from build123d import *

# Parameters (mm, degrees)
F1_DEPTH = 2.54
F2_W     = 10.16
F2_H     = 10.16
F3_DEPTH = 2.54


with BuildPart() as f1:
    # F0 (on Top) → F1 (new body)
    with BuildSketch(Plane.XY):
        with BuildLine():
            Line((206.375, -73.81875), (206.375, 73.81875))
            ThreePointArc((206.375, 73.81875), (196.145704, 98.514454), (171.45, 108.74375))
            Line((171.45, 108.74375), (-171.45, 108.74375))
            ThreePointArc((-171.45, 108.74375), (-196.145704, 98.514454), (-206.375, 73.81875))
            Line((-206.375, 73.81875), (-206.375, -73.81875))
            ThreePointArc((-206.375, -73.81875), (-196.145704, -98.514454), (-171.45, -108.74375))
            Line((-171.45, -108.74375), (171.45, -108.74375))
            ThreePointArc((171.45, -108.74375), (196.145704, -98.514454), (206.375, -73.81875))
        make_face()
        with BuildLine():
            ThreePointArc((187.325, -73.81875), (182.67532, -85.04407), (171.45, -89.69375))
            Line((171.45, -89.69375), (-171.45, -89.69375))
            ThreePointArc((-171.45, -89.69375), (-182.67532, -85.04407), (-187.325, -73.81875))
            Line((-187.325, -73.81875), (-187.325, 73.81875))
            ThreePointArc((-187.325, 73.81875), (-182.67532, 85.04407), (-171.45, 89.69375))
            Line((-171.45, 89.69375), (171.45, 89.69375))
            ThreePointArc((171.45, 89.69375), (182.67532, 85.04407), (187.325, 73.81875))
            Line((187.325, 73.81875), (187.325, -73.81875))
        make_face(mode=Mode.SUBTRACT)
    extrude(amount=F1_DEPTH)

    # F2 (on face) → F3 (cut, through all)
    with BuildSketch(Plane.XY.offset(2.54)):
        with Locations((-131.445, 94.77375)):
            Rectangle(F2_W, F2_H)
        with Locations((114.6175, 94.77375)):
            Rectangle(F2_W, F2_H)
    extrude(amount=-F3_DEPTH, mode=Mode.SUBTRACT)


solid = f1.part
Geometry: final body of the model. Coordinates: model frame, mm. A direction names the side the tool comes from. Round coordinates to 2 decimals unless told otherwise and drop trailing zeros. Loops run counter-clockwise (first coordinate to the right, second up) from the corner with the lowest first, then second, coordinate; pieces in that order, holes last. Notation, with made-up numbers: M 78,19 L 131,19 A12 ccw 131,41 Z; hole C -23,13.5 d1. An arc over 180 degrees is marked long. Put each result on its own line as item: value. Start each with the question number.
(1) Set-up query: faces 1 (the face through (-182.8, 84.92, 1.25)), 2 (the face through (196.416, 98.241, 1.252)). Return all of +Z, -Z, +X, -X, +Y, -Y with unobstructed straight access to the full face (end or side cutting, diameter ignored); none if empty.
(2) Material intervals for line 1 along Y through (x, z) = (-38, 1.05); line 2 along X through (y, z) = (42.5, 1.8) (3 decimals); line 3 along Y through (x, z) = (113, 0.6), sorted ascending. Write a range as [from, to].
(3) Draft query along Y for faces 3 (the face through (-182.55, -85.17, 1.25)), 4 (the face through (195.873, -98.784, 1.252)), 5 (the face through (-1, -96, 2.54)). Return one class per face: +Y half, -Y half, draft (parallel to the pull), parting line (faces both ways), or undercut.
(4) Section query A-A (x = -84). Return loops of the section in (y, z).
(5) Section query B-B (y = 21.5). Return loops of the section in (x, z) (3 decimals).
(6) Contact query for flat-ended pins moving along their axis: pin 1 Ø1.3 at (y, z) = (95, 1.5) entering from -X; pin 2 Ø1.3 at (y, z) = (95, 2) entering from +X. Output: stop coordinate, or through.
Findings below:
1. face 1: +Z, -Z
1. face 2: +Z, -Z, +X, +Y
2. line 1: y = [-108.74, -89.69], [89.69, 108.74]
2. line 2: x = [-206.375, -187.325], [187.325, 206.375]
2. line 3: y = [-108.74, -89.69], [99.85, 108.74]
3. face 3: undercut
3. face 4: -Y half
3. face 5: draft
4. outline: M -108.74,0 L -89.69,0 L -89.69,2.54 L -108.74,2.54 Z; M 89.69,0 L 108.74,0 L 108.74,2.54 L 89.69,2.54 Z
5. outline: M -206.375,0 L -187.325,0 L -187.325,2.54 L -206.375,2.54 Z; M 187.325,0 L 206.375,0 L 206.375,2.54 L 187.325,2.54 Z
6. pin 1: stops at x = -199.7
6. pin 2: stops at x = 199.7
